For this review, take the finished solid that the model builds, in its own axes (mm). Coordinates: 2 decimals unless noted, no trailing zeros. Write each loop counter-clockwise with the first axis right and the second up, starting at its lowest first coordinate (ties: lowest second). Pieces come first, ordered by that corner, then holes.
1) To check wall thickness, follow line 1 along X through (y, z) = (5.25, 0); line 2 along X through (y, z) = (6.75, -126.5); line 3 along Z through (x, y) = (-276, 0.5). State the ranges of each line that lie inside material, in increasing order.
2) We need section A-A on x = 33.5. Write out the cut boundary in (y, z), then the cut area to 3 significant figures.
3) We need section B-B on z = 62. Give the number of separate pieces and of enclosed holes in the cut face, then the cut area to 3 significant figures.
from build123d import *

# Parameters (mm, degrees)
CROQUIS1_W              = 720
CROQUIS1_H              = 340
SALIENTE_EXTRUIR1_DEPTH = 10
CROQUIS3_RX             = 99.333174073
CROQUIS3_RY             = 8.979269973
CROQUIS3_W              = 660
CROQUIS3_H              = 300
CORTAR_EXTRUIR2_DEPTH   = 10


with BuildPart() as part:
    # Croquis1 → Saliente-Extruir1 (new body)
    with BuildSketch(Plane(origin=(0, 0, 0), x_dir=(1, 0, 0), z_dir=(0, 1, 0))):
        Rectangle(CROQUIS1_W, CROQUIS1_H)
    extrude(amount=SALIENTE_EXTRUIR1_DEPTH)

    # Croquis3 → Cortar-Extruir2 (cut)
    with BuildSketch(Plane(origin=(0, 10, 0), x_dir=(1, 0, 0), z_dir=(0, 1, 0))):
        with Locations(Location((-340.089850217, 0), (0, 0, 90))):
            Ellipse(CROQUIS3_RX, CROQUIS3_RY)
        with Locations((10, 0)):
            Rectangle(CROQUIS3_W, CROQUIS3_H)
    extrude(amount=-CORTAR_EXTRUIR2_DEPTH, mode=Mode.SUBTRACT)


solid = part.part
Result:
1. line 1: x = -360 to -349.07, -331.11 to -320, 340 to 360
1. line 2: x = -360 to -320, 340 to 360
1. line 3: z = -170 to -150, 150 to 170
2. outline: (0, -170) - (10, -170) - (10, -150) - (0, -150) - close; (0, 150) - (10, 150) - (10, 170) - (0, 170) - close
2. area: 400 mm2
3. separate pieces: 3
3. enclosed holes: 0
3. area: 460 mm2
